from build123d import *

# Parameters (mm, degrees)
F1_DEPTH = 2
F3_DEPTH = 5
F5_DEPTH = 5


with BuildPart() as f1:
    # F0 (on Top) → F1 (new body)
    with BuildSketch(Plane.XY):
        with BuildLine():
            Line((-15, 5), (-50, 0))
            Line((-50, 0), (0, 0))
            ThreePointArc((0, 0), (2.5, 2.5), (0, 5))
            Line((0, 5), (-15, 5))
        make_face()
    extrude(amount=F1_DEPTH)

    # F2 (on face) → F3 (cut)
    with BuildSketch(Plane.XZ):
        Polygon((-50, 2), (-50, 0), (-12.168623, 2), align=None)
    extrude(amount=-F3_DEPTH, mode=Mode.SUBTRACT)

    # F4 (on face) → F5 (cut)
    with BuildSketch(Plane.XZ):
        Polygon((-9.615218, 2), (-11.471676, 2), (-10.602703, 1.073664), align=None)
        Polygon((-7.615218, 2), (-9.471676, 2), (-8.602703, 1.073664), align=None)
        Polygon((-5.615218, 2), (-7.471676, 2), (-6.602703, 1.073664), align=None)
        Polygon((-3.615218, 2), (-5.471676, 2), (-4.602703, 1.073664), align=None)
        Polygon((-2.602703, 1.073664), (-1.615218, 2), (-3.471676, 2), align=None)
        Polygon((-0.602703, 1.073664), (0, 1.639045), (0, 2), (-1.471676, 2), align=None)
    extrude(amount=-F5_DEPTH, mode=Mode.SUBTRACT)


solid = f1.part
Source: CAD feature listing. Evaluate the final solid. Frame: model axes, mm. A direction names the side the tool comes from. Coordinates: 2 decimals unless noted, no trailing zeros. Order: outer loops, then holes, each group sorted by start corner. A loop starts at its lowest first (then second) coordinate and runs counter-clockwise, first axis right, second up. Notation, with made-up numbers: M -22.75,-30 L 32.25,-30 A17 cw 32.25,-10 Z; hole C 22,18.25 d6. An arc over 180 degrees is marked long. Write each question's results on one line, items separated by ' | '. Start each with the question number.
Item 1: Set-up query: faces 1 (the face through (-28.37, 3.09, 0.71)), 2 (the face through (-5, 2.5, 1.5)). Return all of +Z, -Z, +X, -X, +Y, -Y with unobstructed straight access to the full face (end or side cutting, diameter ignored); none if empty.
Item 2: Cut plane B-B (z = 0.5). Return loops of the section in (x, y), and give its area (3 significant figures).
Item 3: Cut plane A-A (y = 1.3). Return loops of the section in (x, z), and give its area (3 significant figures).
Item 4: First-contact query: pin 1 Ø1.5 at (x, y) = (-34.5, 4.5) entering from +Z. Flat tip, straight axial feed; report the tip coordinate or a pass-through.
Item 5: Cut plane D-D (y = 3.7). Return loops of the section in (x, z), and give its area (3 significant figures).
Item 6: Line query: probe 1 along Z at (x, y) = (-2, 3.1); probe 2 along Z at (x, y) = (-3, 3.25); probe 3 along Y at (x, z) = (-19.5, 1.05). Output: solid intervals per line, ascending.
Item 7: Draft query along X for faces 3 (the face through (-27.146, 1.909, 1.208)), 4 (the face through (-8.116, 2.465, 1.53)), 5 (the face through (-1, 2.5, 1.5)), 6 (the face through (-7, 5, 1)). Return one class per face: pulls with the +X half, pulls with the -X half, needs draft (parallel to the pull), parting line crosses it, or undercut.
Item 8: Cut plane C-C (x = -22.5). Return loops of the section in (y, z), and give its area (3 significant figures).
Checked values:
1) face 1: +Z, -Z, -X, +Y | face 2: +Z, +Y, -Y
2) outline: M -40.54,0 L 0,0 A2.5 ccw 0,5 L -15,5 L -40.54,1.35 Z | area: 166 mm2
3) outline: M -40.9,0 L 2.19,0 L 2.19,2 L 0,2 L 0,1.64 L -0.6,1.07 L -1.47,2 L -1.62,2 L -2.6,1.07 L -3.47,2 L -3.62,2 L -4.6,1.07 L -5.47,2 L -5.62,2 L -6.6,1.07 L -7.47,2 L -7.62,2 L -8.6,1.07 L -9.47,2 L -9.62,2 L -10.6,1.07 L -11.47,2 L -12.17,2 L -40.9,0.48 Z | area: 59.3 mm2
4) pin 1: passes through
5) outline: M -24.1,0 L 2.19,0 L 2.19,2 L 0,2 L 0,1.64 L -0.6,1.07 L -1.47,2 L -1.62,2 L -2.6,1.07 L -3.47,2 L -3.62,2 L -4.6,1.07 L -5.47,2 L -5.62,2 L -6.6,1.07 L -7.47,2 L -7.62,2 L -8.6,1.07 L -9.47,2 L -9.62,2 L -10.6,1.07 L -11.47,2 L -12.17,2 L -24.1,1.37 Z | area: 43.7 mm2
6) probe 1: z = 0 to 1.64 | probe 2: z = 0 to 1.5 | probe 3: y = 0 to 4.36
7) face 3: pulls with the -X half | face 4: undercut | face 5: undercut | face 6: needs draft
8) outline: M 0,0 L 3.93,0 L 3.93,1.45 L 0,1.45 Z | area: 5.71 mm2
